Geometry check sheet. Reference: drawing and pictorial views, mm from the part's lowest x, y, z. A direction names the side the tool comes from. Give positions to 0.01 mm unless a question says otherwise; leave off trailing zeros. Order: outer loops, then holes, each group sorted by start corner. A loop starts at its lowest first (then second) coordinate and runs counter-clockwise, first axis right, second up. Notation, with made-up numbers: (36, -30.75) - (61, -30.75) arc R33 cw to (61, 6.25) - close; hole circle Ø3 at (63.5, -27). An arc over 180 degrees is marked (long way). Answer in a Markdown table with one row per item.
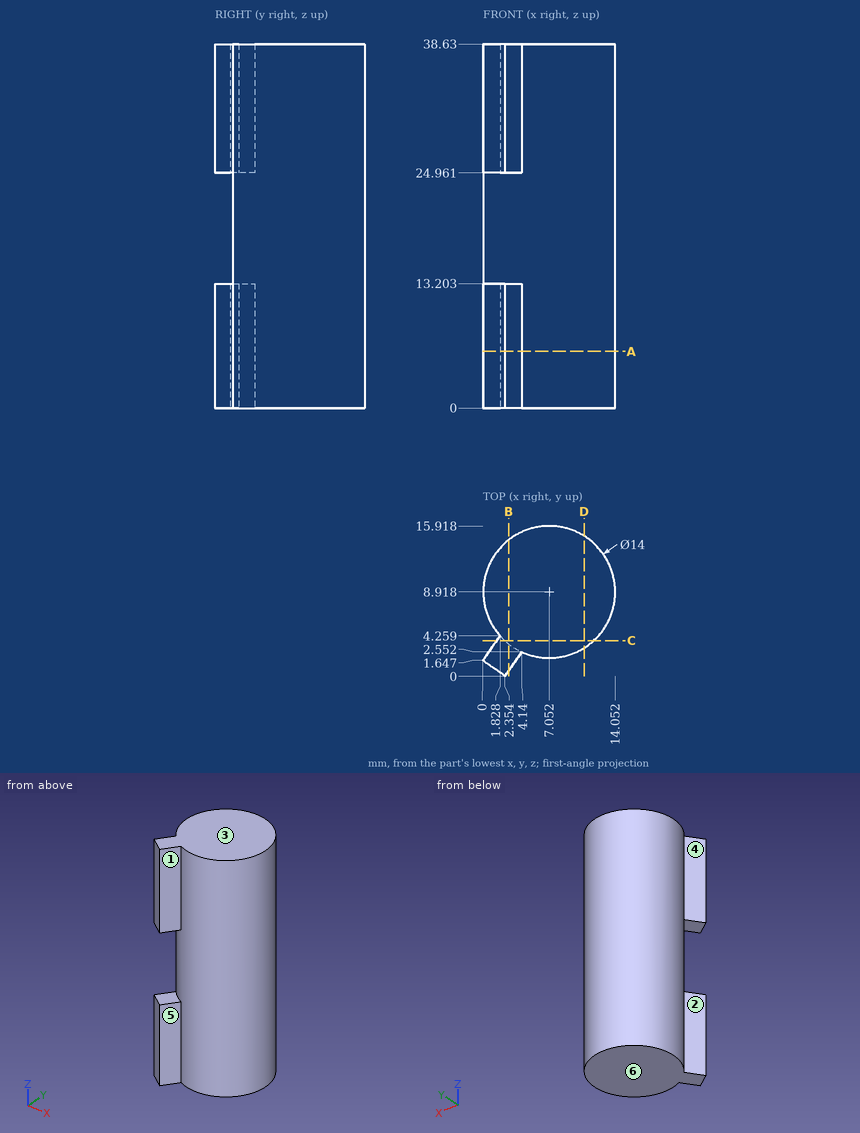
(1) Gauge pin test, flat ends, axial feed: P1, Ø3, axis at y = 12, z = 4, coming from the -X side; P2, Ø5, axis at y = 13.5, z = 22.5, coming from the -X side; P3, Ø1, axis at x = 6.5, z = 15, coming from the +Y side; P4, Ø4, axis at y = 3, z = 31, coming from the -X side. Record the tip position at first contact, or that the pin passes through.
Geometry says:
| item | result |
|---|---|
| P1 | x = 0.23 |
| P2 | x = 0.37 |
| P3 | y = 15.92 |
| P4 | x = 0 |
(2) Cross-section at D-D, the plane x = 10.75. Record the cut outline in (y, z) (1 decimal), then the cut area to 3 significant figures.
Geometry says:
| item | result |
|---|---|
| outline | (3, 0) - (14.9, 0) - (14.9, 38.6) - (3, 38.6) - close |
| area | 459 mm² |
(3) Cross-section at C-C, the plane y = 3.75. Record the cut outline in (x, z), then the cut area to 3 significant figures.
Geometry says:
| item | result |
|---|---|
| outline | (1.47, 0) - (11.77, 0) - (11.77, 38.63) - (1.47, 38.63) - (1.47, 24.96) - (2.33, 24.96) - (2.33, 13.2) - (1.47, 13.2) - close |
| area | 388 mm² |
(4) Thickness scan on L1, parallel to X at y = 15, z = 2 (1 decimal); L2, parallel to X at y = 7, z = 33 (1 decimal); L3, parallel to Y at x = 4.5, z = 24 (1 decimal). Record the ranges inside material, lowest first.
Geometry says:
| item | result |
|---|---|
| L1 | 3.6 to 10.5 |
| L2 | 0.3 to 13.8 |
| L3 | 2.4 to 15.4 |
(5) Cross-section at A-A, the plane z = 6. Record the cut outline in (x, y).
Geometry says:
| item | result |
|---|---|
| outline | (0, 1.65) - (2.35, 0) - (4.14, 2.55) arc R7 ccw (long way) to (1.83, 4.26) - close |
(6) Cross-section at B-B, the plane x = 2.75. Record the cut outline in (y, z) (1 decimal), then the cut area to 3 significant figures.
Geometry says:
| item | result |
|---|---|
| outline | (0.6, 0) - (14.4, 0) - (14.4, 38.6) - (0.6, 38.6) - (0.6, 25) - (3.4, 25) - (3.4, 13.2) - (0.6, 13.2) - close |
| area | 503 mm² |
(7) Mould release check, pull along Y, two halves, no side actions. Record for the marked faces 1, 2, 3 and 4: pulls with the +Y half, pulls with the -Y half, needs draft (parallel to the pull), parting line crosses it, or undercut.
Geometry says:
| item | result |
|---|---|
| face 1 | pulls with the -Y half |
| face 2 | undercut |
| face 3 | needs draft |
| face 4 | undercut |
(8) Access from +Z, -Z, +X, -X, +Y, -Y to the whole of each face (thin tool, end or side, straight path). Record for the marked faces 5 and 6.
Geometry says:
| item | result |
|---|---|
| face 5 | +Z, -Z, -Y |
| face 6 | -Z, +X, -X, +Y, -Y |
